from build123d import *

# Parameters (mm, degrees)
SKETCH_1_R                = 26
EXTRUDE_1_DEPTH           = 5
SKETCH_2_R                = 14
CUT_EXTRUDE_1_DEPTH       = 7
SKETCH_3_R                = 10
CUT_EXTRUDE_2_DEPTH       = 38.429934544
HOLE_WIZARD_1_D           = 5.5
HOLE_WIZARD_1_CBORE_D     = 10
HOLE_WIZARD_1_CBORE_DEPTH = 5.7
CHAMFER_1_SIZE            = 0.5
PATTERN_CIRCULAR_1_COUNT  = 3


with BuildPart() as part:
    # 草图1 → 凸台-拉伸1 (new, symmetric)
    with BuildSketch(Plane.XY):
        Circle(SKETCH_1_R)
    extrude(amount=EXTRUDE_1_DEPTH, both=True)

    # 草图2 → 切除-拉伸1 (cut)
    with BuildSketch(Plane.XY.offset(5)):
        Circle(SKETCH_2_R)
    extrude(amount=-CUT_EXTRUDE_1_DEPTH, mode=Mode.SUBTRACT)

    # 草图3 → 切除-拉伸2 (cut, through all)
    with BuildSketch(Plane.XY.offset(-2)):
        Circle(SKETCH_3_R)
    extrude(amount=-CUT_EXTRUDE_2_DEPTH, mode=Mode.SUBTRACT)

    # 打孔尺寸根据内六角圆柱头螺钉的类型1 (through all)
    with Locations(Plane.XY.offset(5)):
        with Locations((0, 20)):
            hole_wizard_1 = CounterBoreHole(HOLE_WIZARD_1_D / 2, HOLE_WIZARD_1_CBORE_D / 2, HOLE_WIZARD_1_CBORE_DEPTH)

    # 倒角1
    chamfer_1_edges = [part.edges().sort_by_distance(p)[0] for p in [
        (-26, 0, -5),
        (-26, 0, 5),
    ]]
    chamfer(chamfer_1_edges, length=CHAMFER_1_SIZE)

    # 阵列(圆周)1: 打孔尺寸根据内六角圆柱头螺钉的类型1 ×3 about axis
    pattern_circular_1_axis = Axis((0, 0, 0), (0, 0, 1))
    for i in range(1, PATTERN_CIRCULAR_1_COUNT):
        add(hole_wizard_1.rotate(pattern_circular_1_axis, i * 360 / PATTERN_CIRCULAR_1_COUNT), mode=Mode.SUBTRACT)


solid = part.part
Can you work these out from the model? Positions are in its coordinate system, mm. A direction names the side the tool comes from. Coordinates: 2 decimals unless noted, no trailing zeros. Order: outer loops, then holes, each group sorted by start corner. A loop starts at its lowest first (then second) coordinate and runs counter-clockwise, first axis right, second up. Notation, with made-up numbers: M 78,-23.75 L 93,-23.75 A20 ccw 93,-19.75 Z; hole C 18,23.25 d6. An arc over 180 degrees is marked long. Write item = value, one per line.
(1) For pin 1 Ø6.5 at (x, y) = (-17.32, -10) entering from -Z; pin 2 Ø3.5 at (x, y) = (0, 20) entering from +Z; pin 3 Ø25 at (x, y) = (0, 0) entering from +Z; pin 4 Ø2 at (y, z) = (17.5, 0.5) entering from +X, each with a flat end and sliding along its axis, tell me the tip position at first contact or that it passes through.
Results are:
pin_1 = -5
pin_2 = through
pin_3 = -2
pin_4 = 20.09
(2) Suppose I cut it at D-D on y = -9. State how many separate pieces and enclosed holes the cut face has, plus the area to 3 significant figures.
Results are:
separate_pieces = 4
enclosed_holes = 0
area = 155 mm2
(3) I need wall thicknesses on line 1 along Y through (x, z) = (0, -3.7); line 2 along X through (y, z) = (-14.5, 0.25); line 3 along Y through (x, z) = (-2.5, 1). Which ranges of each line are inside material? Lowest first, please. Write a range as [from, to].
Results are:
line_1 = [-26, -10], [10, 17.25], [22.75, 26]
line_2 = [-21.58, -19.5], [-15.14, 15.14], [19.5, 21.58]
line_3 = [-25.88, -13.77], [13.77, 15.67], [24.33, 25.88]
(4) Suppose I cut it at B-B on y = 0. Please give me the cut outline in (x, z).
Results are:
outline = M -26,-4.5 L -25.5,-5 L -10,-5 L -10,-2 L -14,-2 L -14,5 L -25.5,5 L -26,4.5 Z; M 10,-5 L 25.5,-5 L 26,-4.5 L 26,4.5 L 25.5,5 L 14,5 L 14,-2 L 10,-2 Z
(5) If we mould it in two halves opening along Y, with no side actions, what happens to faces 3 (the face through (11, -11, 5)), 4 (the face through (-20.633, -15.821, 0.063)), 5 (the face through (-3, 10, -2))? For each: pulls with the +Y half, pulls with the -Y half, needs draft (parallel to the pull), parting line crosses it, or undercut.
Results are:
face_3 = needs draft
face_4 = parting line crosses it
face_5 = undercut
(6) Suppose I cut it at A-A on x = 0. Please give me the cut outline in (y, z), plus the area to 3 significant figures.
Results are:
outline = M -26,-4.5 L -25.5,-5 L -10,-5 L -10,-2 L -14,-2 L -14,5 L -25.5,5 L -26,4.5 Z; M 10,-5 L 17.25,-5 L 17.25,-0.7 L 15,-0.7 L 15,5 L 14,5 L 14,-2 L 10,-2 Z; M 22.75,-5 L 25.5,-5 L 26,-4.5 L 26,4.5 L 25.5,5 L 25,5 L 25,-0.7 L 22.75,-0.7 Z
area = 183 mm2
(7) Suppose I cut it at C-C on z = 1. Please give me the cut outline in (x, y).
Results are:
outline = C 0,0 d52; hole C -17.32,-10 d10; hole C 0,0 d28; hole C 0,20 d10; hole C 17.32,-10 d10
(8) For faces 1 (the face through (-12.702, -11.915, 2.19)), 2 (the face through (-2.17, -9.76, -3.48)), which set-ups out of +Z, -Z, +X, -X, +Y, -Y let a thin tool reach every point of the face, with its end or its side?
Results are:
face_1 = +Z
face_2 = +Z, -Z
